```python
from build123d import *

# Parameters (mm, degrees)
SKETCH1_W           = 304.8
SKETCH1_H           = 304.8
BOSS_EXTRUDE1_DEPTH = 3.175


with BuildPart() as part:
    # Sketch1 → Boss-Extrude1 (new body)
    with BuildSketch(Plane(origin=(0, 0, 0), x_dir=(1, 0, 0), z_dir=(0, 1, 0))):
        with Locations((-12.540052417, 0)):
            Rectangle(SKETCH1_W, SKETCH1_H)
        Polygon((-75.698500695, 63.659947583), (-25.559947583, 63.659947583), (-25.559947583, 108.120227238), (-31.557978093, 114.118257748), (-75.698500695, 114.118257748), align=None, mode=Mode.SUBTRACT)
        Polygon((38.701669621, 63.703874457), (88.840222733, 63.703874457), (88.840222733, 108.164154112), (82.842192224, 114.162184621), (38.701669621, 114.162184621), align=None, mode=Mode.SUBTRACT)
        Polygon((-75.76813518, -25.114152208), (-25.629582068, -25.114152208), (-25.629582068, 19.346127447), (-31.627612577, 25.344157957), (-75.76813518, 25.344157957), align=None, mode=Mode.SUBTRACT)
        Polygon((38.837246674, -25.31385175), (88.975799786, -25.31385175), (88.975799786, 19.146427905), (82.977769277, 25.144458414), (38.837246674, 25.144458414), align=None, mode=Mode.SUBTRACT)
        Polygon((38.618131254, -113.973933449), (88.756684366, -113.973933449), (88.756684366, -69.513653793), (82.758653857, -63.515623284), (38.618131254, -63.515623284), align=None, mode=Mode.SUBTRACT)
        Polygon((-75.926077633, -113.955197726), (-25.787524521, -113.955197726), (-25.787524521, -69.494918071), (-31.78555503, -63.496887561), (-75.926077633, -63.496887561), align=None, mode=Mode.SUBTRACT)
    extrude(amount=BOSS_EXTRUDE1_DEPTH)


solid = part.part
```
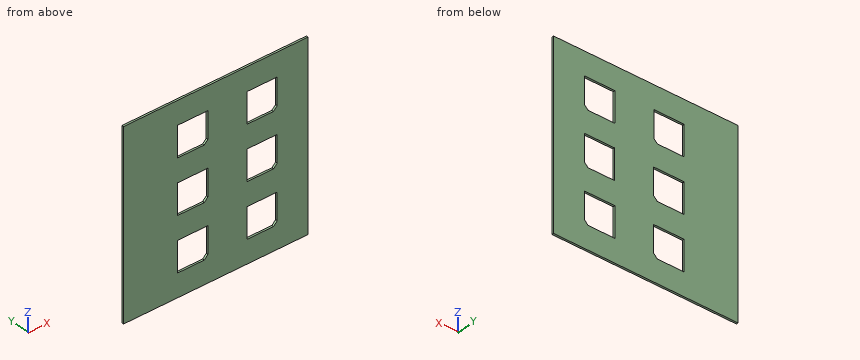
Design review of the part built by this model. Coordinates are the model's own, in mm. Coordinates: 2 decimals unless noted, no trailing zeros. Order: outer loops, then holes, each group sorted by start corner. A loop starts at its lowest first (then second) coordinate and runs counter-clockwise, first axis right, second up.
1) Clearance check with a flat-ended pin moving along its axis: pin 1 (12 mm diameter, centred on x = 109, z = 68.5, fed in from -Y). State where the tip first meets the part, or that it passes through.
2) Take a section at B-B, the plane y = 1.95. State how many separate pieces and enclosed holes the cut face has, and give its area (3 significant figures).
3) Wall thickness on line 1 along X through (y, z) = (1.9, -17); line 2 along Z through (x, y) = (53, 2.25); line 3 along Z through (x, y) = (-45, 2.65): over which ranges is each line inside the solid? List them lowest first.
4) Take a section at C-C, the plane z = 75. Give the boundary of the cut face in (x, y) (3 decimals).
5) Take a section at A-A, the plane x = 76. Give the boundary of the cut face in (y, z) (3 decimals).
Returned:
1. pin 1: stops at y = 0
2. separate pieces: 1
2. enclosed holes: 6
2. area: 77,800 mm2
3. line 1: x = -164.94 to -75.77, -25.63 to 38.84, 88.98 to 139.86
3. line 2: z = -152.4 to -114.16, -63.7 to -25.14, 25.31 to 63.52, 113.97 to 152.4
3. line 3: z = -152.4 to -114.12, -63.66 to -25.34, 25.11 to 63.5, 113.96 to 152.4
4. outline: (-164.94, 0) - (-75.926, 0) - (-75.926, 3.175) - (-164.94, 3.175) - close; (-25.788, 0) - (38.618, 0) - (38.618, 3.175) - (-25.788, 3.175) - close; (88.757, 0) - (139.86, 0) - (139.86, 3.175) - (88.757, 3.175) - close
5. outline: (0, -152.4) - (3.175, -152.4) - (3.175, -114.162) - (0, -114.162) - close; (0, -63.704) - (3.175, -63.704) - (3.175, -25.144) - (0, -25.144) - close; (0, 25.314) - (3.175, 25.314) - (3.175, 63.516) - (0, 63.516) - close; (0, 113.974) - (3.175, 113.974) - (3.175, 152.4) - (0, 152.4) - close
